Geometry: final body of the model. Coordinates: model frame, mm. Give positions to 0.01 mm unless a question says otherwise; leave off trailing zeros. Write each loop counter-clockwise with the first axis right and the second up, starting at its lowest first coordinate (ties: lowest second). Pieces come first, ordered by that corner, then holes. Notation, with made-up numbers: (65, 37.5) - (120, 37.5) arc R9 ccw to (120, 51.5) - close; hole circle Ø3 at (23, 59). An arc over 180 degrees is marked (long way). Return JSON: item names as keys, results as strings.
from build123d import *

# Parameters (mm, degrees)
F0_W     = 7.05
F0_H     = 3.5
F1_DEPTH = 11.2
F3_D     = 2.38
F3_DEPTH = 3.25
F3_TIP   = 0.7150241366
F5_D     = 1.3
F8_DEPTH = 3.25


with BuildPart() as f1:
    # F0 (on Top) → F1 (new body)
    with BuildSketch(Plane.XY):
        Rectangle(F0_W, F0_H)
        with BuildLine():
            ThreePointArc((-3.525, 1.75), (-5.275, 0), (-3.525, -1.75))
            Line((-3.525, -1.75), (-3.525, 1.75))
        make_face()
    extrude(amount=F1_DEPTH)

    # F3
    with Locations(Plane.XY.offset(11.2)):
        with Locations((-0.725, 0)):
            Hole(F3_D / 2, depth=F3_DEPTH)
            with Locations((0, 0, -(F3_DEPTH + F3_TIP / 2))):  # 118° drill point
                Cone(0, F3_D / 2, F3_TIP, mode=Mode.SUBTRACT)

    # F5 (through all)
    with Locations(Plane.XY.offset(11.2)):
        with Locations((-3.525, 0), (-0.725, 0), (2.075, 0)):
            Hole(F5_D / 2)

    # F7 (on face) → F8 (cut)
    with BuildSketch(Plane.XY.offset(11.2)):
        with BuildLine():
            Line((-1.6765881673, -1.75), (0.3234118327, -1.75))
            Line((0.3234118327, -1.75), (0.3234118327, -0.562967698))
            ThreePointArc((0.3234118327, -0.562967698), (-0.6350671823, -1.1865968516), (-1.6765881673, -0.7145487806))
            Line((-1.6765881673, -0.7145487806), (-1.6765881673, -1.75))
        make_face()
        with BuildLine():
            ThreePointArc((-1.6765881673, 0.7145487806), (-0.6350671823, 1.1865968516), (0.3234118327, 0.562967698))
            Line((0.3234118327, 0.562967698), (0.3234118327, 1.75))
            Line((0.3234118327, 1.75), (-1.6765881673, 1.75))
            Line((-1.6765881673, 1.75), (-1.6765881673, 0.7145487806))
        make_face()
    extrude(amount=-F8_DEPTH, mode=Mode.SUBTRACT)


solid = f1.part
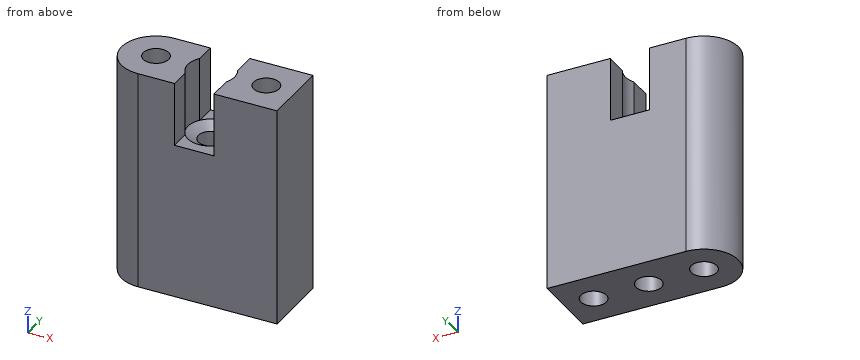
Q1. Pin query (flat end, axial travel): P1, Ø1, axis at x = 2.075, y = 0, coming from the +Z side; P2, Ø0.6, axis at x = -0.5, y = -1.5, coming from the +Z side; P3, Ø1.3, axis at y = 1, z = 10.5, coming from the -X side; P4, Ø0.6, axis at y = -1, z = 9, coming from the -X side. Return the tip coordinate at first contact, or that it passes through.
Answer key:
{"P1": "passes through", "P2": "stops at z = 7.95", "P3": "stops at x = -5.24", "P4": "stops at x = -5.13"}
Q2. Material intervals for probe 1 along Y at (x, z) = (1.75, 1.5); probe 2 along X at (y, z) = (0.2, 9.5) (3 decimals); probe 3 along Y at (x, z) = (1.5, 3), sorted ascending. Write a range as [from, to].
Answer key:
{"probe 1": "y = [-1.75, -0.56], [0.56, 1.75]", "probe 2": "x = [-5.264, -4.143], [-2.907, -1.898], [0.448, 1.457], [2.693, 3.525]", "probe 3": "y = [-1.75, -0.3], [0.3, 1.75]"}
Q3. Section query D-D, the plane x = 1.75. Return the cut outline in (y, z).
Answer key:
{"outline": "(-1.75, 0) - (-0.56, 0) - (-0.56, 11.2) - (-1.75, 11.2) - close; (0.56, 0) - (1.75, 0) - (1.75, 11.2) - (0.56, 11.2) - close"}
Q4. Section query C-C, the plane z = 2. Return the cut outline in (x, y) (3 decimals).
Answer key:
{"outline": "(-3.525, -1.75) - (3.525, -1.75) - (3.525, 1.75) - (-3.525, 1.75) arc R1.75 ccw to start; hole circle Ø1.3 at (-3.525, 0); hole circle Ø1.3 at (-0.725, 0); hole circle Ø1.3 at (2.075, 0)"}
Q5. Section query B-B, the plane y = 0. Return the cut outline in (x, z) (3 decimals), plus the area to 3 significant figures.
Answer key:
{"outline": "(-5.275, 0) - (-4.175, 0) - (-4.175, 11.2) - (-5.275, 11.2) - close; (-2.875, 0) - (-1.375, 0) - (-1.375, 7.626) - (-1.915, 7.95) - (-1.915, 11.2) - (-2.875, 11.2) - close; (-0.075, 0) - (1.425, 0) - (1.425, 11.2) - (0.465, 11.2) - (0.465, 7.95) - (-0.075, 7.626) - close; (2.725, 0) - (3.525, 0) - (3.525, 11.2) - (2.725, 11.2) - close", "area": "51.2 mm^2"}
Q6. Section query A-A, the plane z = 9.5. Return the cut outline in (x, y) (3 decimals), plus the area to 3 significant figures.
Answer key:
{"outline": "(-3.525, -1.75) - (-1.677, -1.75) - (-1.677, -0.715) arc R1.19 cw to (-1.677, 0.715) - (-1.677, 1.75) - (-3.525, 1.75) arc R1.75 ccw to start; (0.323, -1.75) - (3.525, -1.75) - (3.525, 1.75) - (0.323, 1.75) - (0.323, 0.563) arc R1.19 cw to (0.323, -0.563) - close; hole circle Ø1.3 at (-3.525, 0); hole circle Ø1.3 at (2.075, 0)", "area": "19.5 mm^2"}
